```python
from build123d import *

# Parameters (mm, degrees)
F0_R          = 16.51
F1_DEPTH      = 152.4
F1_DEPTH_BACK = 152.4
F2_R          = 16.51
F3_DEPTH      = 152.4
F5_R          = 16.51
F6_DEPTH      = 152.4
F7_R          = 15.875
F8_DEPTH      = 304.801
F9_R          = 15.875
F10_DEPTH     = 152.41
F11_R         = 15.875
F12_DEPTH     = 152.41
F13_R         = 16.51
F14_DEPTH     = 135.89
F15_R         = 16.51
F16_DEPTH     = 1.27


with BuildPart() as f1:
    # F0 (on Front) → F1 (new body, two sides)
    with BuildSketch(Plane.XZ) as f1_sk:
        Circle(F0_R)
    extrude(amount=F1_DEPTH)
    extrude(f1_sk.sketch, amount=-F1_DEPTH_BACK)

    # F2 (on Right) → F3 (join)
    with BuildSketch(Plane.YZ):
        Circle(F2_R)
    extrude(amount=F3_DEPTH)

    # F5 (on face) → F6 (join)
    with BuildSketch(Plane(origin=(0, 0, 0), x_dir=(0, 1, 0), z_dir=(0.7071067812, 0, 0.7071067812))):
        Circle(F5_R)
    extrude(amount=-F6_DEPTH)

    # F7 (on face) → F8 (cut, through all)
    with BuildSketch(Plane.XZ.offset(152.4)):
        Circle(F7_R)
    extrude(amount=-F8_DEPTH, mode=Mode.SUBTRACT)

    # F9 (on face) → F10 (cut, up to face)
    with BuildSketch(Plane.YZ.offset(152.4)):
        Circle(F9_R)
    extrude(amount=-F10_DEPTH, mode=Mode.SUBTRACT)

    # F11 (on face) → F12 (cut, up to face)
    with BuildSketch(Plane(origin=(-107.7630734528, 0, -107.7630734528), x_dir=(0, -1, 0), z_dir=(-0.7071067812, 0, -0.7071067812))):
        Circle(F11_R)
    extrude(amount=-F12_DEPTH, mode=Mode.SUBTRACT)

    # F13 (on face) → F14 (cut)
    with BuildSketch(Plane(origin=(0, 152.4, 0), x_dir=(-1, 0, 0), z_dir=(0, 1, 0))):
        Circle(F13_R)
    extrude(amount=-F14_DEPTH, mode=Mode.SUBTRACT)

    # F15 (on face) → F16 (join)
    with BuildSketch(Plane(origin=(0, 16.51, 0), x_dir=(-1, 0, 0), z_dir=(0, 1, 0))):
        Circle(F15_R)
    extrude(amount=-F16_DEPTH)


solid = f1.part
```
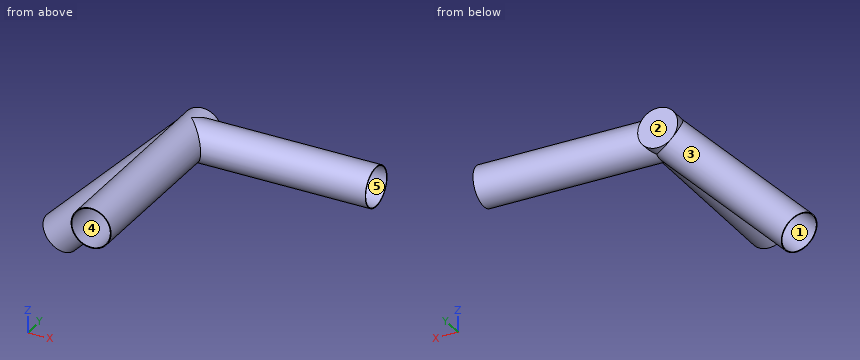
The listing builds one solid part. Answer for the finished solid, in the listing's coordinates (mm). Face numbers are marked on the shaded views. A direction names the side the tool comes from. Coordinates: 2 decimals unless noted, no trailing zeros. Loops run counter-clockwise (first coordinate to the right, second up) from the corner with the lowest first, then second, coordinate; pieces in that order, holes last. Notation, with made-up numbers: (78, 38) -> (108, 38) arc R28 ccw to (108, 70) -> close; hole circle Ø11 at (-22.75, 52). An arc over 180 degrees is marked (long way). Return JSON: item names as keys, results as strings. Group by question number.
(1) Determine the mould class of the marked faces 1 and 2 for opening direction X: released by +X, released by -X, zero draft, split by the parting line, or undercut.
(2) A cutting plane is placed at A-A on y = -58.5. Write down the section's boundary in (x, z) (3 decimals).
(3) Given pin 1 Ø4 at (x, y) = (15, -26.5) entering from +Z; pin 2 Ø9.5 at (x, z) = (3.5, 3) entering from -Y; pin 3 Ø5 at (x, y) = (110, -6) entering from +Z, each flat-ended and moving along its own axis, determine where each tip first touches the part or whether it passes through.
(4) Which of the six approach directions +Z, -Z, +X, -X, +Y, -Y give full straight-line access (tool end or side, diameter ignored) to the marked faces 3, 4 and 5?
(5) Find the intervals of material crossed by probe 1 along Z at (x, y) = (0, -19) (3 decimals); probe 2 along Y at (x, z) = (-54, -55.5), in increasing order. Write a range as from..to.
The answers:
{
 "1": {"face 1": "undercut", "face 2": "zero draft"},
 "2": {"outline": "circle Ø33.02 at (0, 0); hole circle Ø31.75 at (0, 0)"},
 "3": {"pin 1": "stops at z = 10.18", "pin 2": "stops at y = 15.24", "pin 3": "stops at z = 16.13"},
 "4": {"face 3": "none", "face 4": "-Y", "face 5": "+X"},
 "5": {"probe 1": "z = -16.51..-15.875, 15.875..16.51", "probe 2": "y = -16.48..-15.84, 15.84..16.48"}
}
